Check sheet for the modelled part. Datum: model origin and axes. Units: mm. A direction names the side the tool comes from. Round coordinates to 2 decimals unless told otherwise and drop trailing zeros. Write each loop counter-clockwise with the first axis right and the second up, starting at its lowest first coordinate (ties: lowest second). Pieces come first, ordered by that corner, then holes.
from build123d import *

# Parameters (mm, degrees)
F1_DEPTH = 50
F2_R     = 10
F3_R     = 5
F4_DEPTH = 25


# Not quite as in the source:
# - a feature of the source that left no trace in its solid (it failed there, or was rolled back) is left out


with BuildPart() as f1:
    # F0 (on Front) → F1 (new body)
    with BuildSketch(Plane.XZ):
        Polygon((50, 0), (0, 0), (0, -7), (140, -7), (140, 3), (50, 3), align=None)
    extrude(amount=F1_DEPTH)

    # F2
    f2_edges = [f1.edges().sort_by_distance(p)[0] for p in [
        (0, -50, -3.5),
        (0, 0, -3.5),
        (140, 0, -2),
        (140, -50, -2),
    ]]
    fillet(f2_edges, radius=F2_R)

    # F3 (on face) → F4 (cut)
    with BuildSketch(Plane(origin=(0, 0, -7), x_dir=(1, 0, 0), z_dir=(0, 0, -1))):
        with Locations((25, 25)):
            Circle(F3_R)
        with Locations((111.0006011832, 12.5048019411)):
            Circle(F3_R)
    extrude(amount=-F4_DEPTH, mode=Mode.SUBTRACT)


solid = f1.part
1. Go/stop test with flat-tipped pins: pin 1 (15 mm diameter, centred on x = 18.5, y = -29, fed in from +Z); pin 2 (3 mm diameter, centred on y = -44.5, z = -1.5, fed in from +X). Record where each tip stops, or that it passes through.
2. Set-up check for faces 4 (the flat face through (96, -25, 3)), 5 (the flat face through (31, -25, 0)): record each of +Z, -Z, +X, -X, +Y, -Y from which the full face is reachable in a straight line by a thin tool's end or side.
3. Sectioned sample at B-B, the plane x = 25. Enter the section's corners in (y, z).
4. Sectioned sample at C-C, the plane z = -3. Enter the section's corners in (x, y), plus the area to 3 significant figures.
5. Scan lines: line 1 along X through (y, z) = (-25, -3); line 2 along Y through (x, z) = (25, -2.5); line 3 along X through (y, z) = (-24, -0.5). Record each from-to range of solid material in increasing order.
6. Release check for a two-part mould opening along Y. For faces 1 (the flat face through (140, -25, -2)), 2 (the cylindrical face through (137.15, -3.01, -1.93)), 3 (the cylindrical face through (23.92, -20.12, -3.55)) record: released by +Y, released by -Y, zero draft, split by the parting line, or undercut.
7. Sectioned sample at D-D, the plane y = -37.5. Enter the section's corners in (x, z), plus the area to 3 significant figures.
8. Sectioned sample at A-A, the plane y = -25. Enter the section's corners in (x, z).
Computed values:
1. pin 1: stops at z = 0
1. pin 2: stops at x = 139.54
2. face 4: +Z, +X, -X, +Y, -Y
2. face 5: +Z, -X, +Y, -Y
3. outline: (-50, -7) - (-30, -7) - (-30, 0) - (-50, 0) - close; (-20, -7) - (0, -7) - (0, 0) - (-20, 0) - close
4. outline: (0, -40) arc R10 ccw to (10, -50) - (130, -50) arc R10 ccw to (140, -40) - (140, -10) arc R10 ccw to (130, 0) - (10, 0) arc R10 ccw to (0, -10) - close; hole circle Ø10 at (25, -25); hole circle Ø10 at (111, -12.5)
4. area: 6,760 mm2
5. line 1: x = 0 to 20, 30 to 140
5. line 2: y = -50 to -30, -20 to 0
5. line 3: x = 0 to 20.1, 29.9 to 140
6. face 1: zero draft
6. face 2: released by +Y
6. face 3: undercut
7. outline: (0, -7) - (140, -7) - (140, 3) - (50, 3) - (50, 0) - (0, 0) - close
7. area: 1,250 mm2
8. outline: (0, -7) - (20, -7) - (20, 0) - (0, 0) - close; (30, -7) - (140, -7) - (140, 3) - (50, 3) - (50, 0) - (30, 0) - close
